For this review, take the finished solid that the model builds, in its own axes (mm). Coordinates: 2 decimals unless noted, no trailing zeros. Loops run counter-clockwise (first coordinate to the right, second up) from the corner with the lowest first, then second, coordinate; pieces in that order, holes last. Notation, with made-up numbers: M 6.25,75 L 22.25,75 A24 ccw 22.25,95 Z; hole C 78,53.5 d11. An arc over 180 degrees is marked long. Answer as a JSON object with one key per item and string values. Group by question number.
Item 1: Mouldability with a two-part tool opening along Y and no side actions: class faces 1 (the face through (53, 0, 53.975)), 2 (the face through (53, -25.4, 52)), 3 (the face through (114.03, 0.45, 52.37)), 4 (the face through (92.03, 0.45, 52.37)) as +Y half, -Y half, draft (parallel to the pull), parting line (faces both ways), or undercut.
Item 2: Add section A-A (y = 0). State the section outline as (x, z) points (3 decimals).
Item 3: Add section C-C (y = 11). State the section outline as (x, z) points (3 decimals), then the cut area to 3 significant figures.
Item 4: Wall thickness on L1, parallel to Y at x = 90.6, z = 51.45; L2, parallel to X at y = -5.5, z = 51.55; L3, parallel to X at y = 19, z = 53.5: over which ranges is each line inside the solid? List them lowest first. Write a range as from..to.
Item 5: Add section B-B (x = 90.6). State the section outline as (y, z) points (3 decimals), then the cut area to 3 significant figures.
from build123d import *

# Parameters (mm, degrees)
SKETCH1_R           = 3.175
SKETCH1_R_2         = 1.5
BOSS_EXTRUDE1_DEPTH = 3.175


with BuildPart() as part:
    # Sketch1 → Boss-Extrude1 (new body)
    with BuildSketch(Plane.XY.offset(50.8)):
        Polygon((0, 25.4), (-12.7, 25.4), (-12.7, -25.4), (0, -25.4), (120.657586649, -25.4), (120.64241505, 25.4), align=None)
        with Locations((101.6, 0)):
            Circle(SKETCH1_R, mode=Mode.SUBTRACT)
        with Locations((101.6, 11)):
            Circle(SKETCH1_R_2, mode=Mode.SUBTRACT)
        with Locations((112.6, 0)):
            Circle(SKETCH1_R_2, mode=Mode.SUBTRACT)
        with Locations((101.6, -11)):
            Circle(SKETCH1_R_2, mode=Mode.SUBTRACT)
        with Locations((90.6, 0)):
            Circle(SKETCH1_R_2, mode=Mode.SUBTRACT)
    extrude(amount=BOSS_EXTRUDE1_DEPTH)


solid = part.part
From the geometry:
{
 "1": {"face 1": "draft", "face 2": "-Y half", "face 3": "undercut", "face 4": "undercut"},
 "2": {"outline": "M -12.7,50.8 L 89.1,50.8 L 89.1,53.975 L -12.7,53.975 Z; M 92.1,50.8 L 98.425,50.8 L 98.425,53.975 L 92.1,53.975 Z; M 104.775,50.8 L 111.1,50.8 L 111.1,53.975 L 104.775,53.975 Z; M 114.1,50.8 L 120.65,50.8 L 120.65,53.975 L 114.1,53.975 Z"},
 "3": {"outline": "M -12.7,50.8 L 100.1,50.8 L 100.1,53.975 L -12.7,53.975 Z; M 103.1,50.8 L 120.647,50.8 L 120.647,53.975 L 103.1,53.975 Z", "area": "414 mm²"},
 "4": {"L1": "y = -25.4..-1.5, 1.5..25.4", "L2": "x = -12.7..120.65", "L3": "x = -12.7..120.64"},
 "5": {"outline": "M -25.4,50.8 L -1.5,50.8 L -1.5,53.975 L -25.4,53.975 Z; M 1.5,50.8 L 25.4,50.8 L 25.4,53.975 L 1.5,53.975 Z", "area": "152 mm²"}
}
